Can you work these out from the model? Positions are in its coordinate system, mm. Give positions to 0.01 mm unless a question says otherwise; leave off trailing zeros. Order: outer loops, then holes, each group sorted by start corner. A loop starts at its lowest first (then second) coordinate and runs counter-clockwise, first axis right, second up.
Item 1: I want a section at B-B, the plane z = 12. Write out the boundary of the cut face in (x, y), then the cut area to 3 significant figures.
Item 2: I want a section at C-C, the plane y = 1.4. Count the separate pieces of the cut face and the enclosed holes in it, then the cut area to 3 significant figures.
Item 3: If I drill on line 1 along X through (y, z) = (2.1, -27.88); line 2 along X through (y, z) = (3.8, -28.5); line 3 along Z through (x, y) = (26.5, 3.15), over which ranges is the centre line in solid material (lowest first)?
Item 4: I want a section at A-A, the plane x = -2.5. Write out the boundary of the cut face in (y, z).
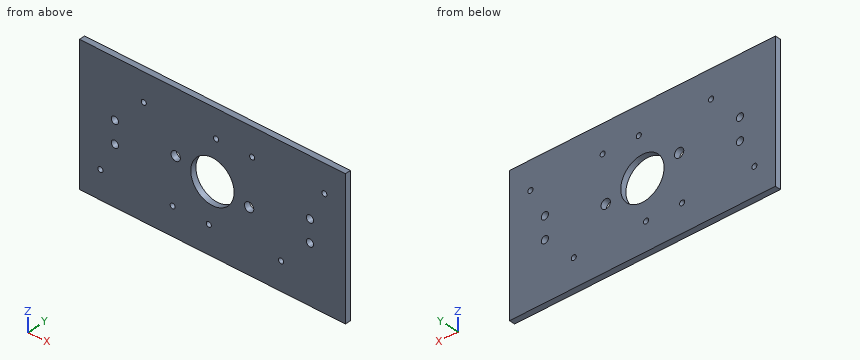
```python
from build123d import *

# Parameters (mm, degrees)
SKETCH1_W           = 184
SKETCH1_H           = 94
SKETCH1_R           = 15
SKETCH1_R_2         = 1.75
SKETCH1_R_3         = 3.225
SKETCH1_R_4         = 2.5
BOSS_EXTRUDE1_DEPTH = 4


with BuildPart() as part:
    # Sketch1 → Boss-Extrude1 (new body)
    with BuildSketch(Plane(origin=(0, 0, 0), x_dir=(1, 0, 0), z_dir=(0, 1, 0))):
        Rectangle(SKETCH1_W, SKETCH1_H)
        with Locations(Location((0, 0, 0), (0, 0, 270))):
            Circle(SKETCH1_R, mode=Mode.SUBTRACT)
        with Locations(Location((-2.5, 27.88, 0), (0, 0, 270))):
            Circle(SKETCH1_R_2, mode=Mode.SUBTRACT)
        with Locations(Location((-27.5, 27.88, 0), (0, 0, 270))):
            Circle(SKETCH1_R_2, mode=Mode.SUBTRACT)
        with Locations(Location((47.5, 27.88, 0), (0, 0, 270))):
            Circle(SKETCH1_R_2, mode=Mode.SUBTRACT)
        with Locations(Location((-77.5, 27.88, 0), (0, 0, 270))):
            Circle(SKETCH1_R_2, mode=Mode.SUBTRACT)
        with Locations(Location((25.4, 4.36, 0), (0, 0, 270))):
            Circle(SKETCH1_R_3, mode=Mode.SUBTRACT)
        with Locations(Location((-67.5, 7.5, 0), (0, 0, 270))):
            Circle(SKETCH1_R_4, mode=Mode.SUBTRACT)
        with Locations(Location((67.5, 7.5, 0), (0, 0, 270))):
            Circle(SKETCH1_R_4, mode=Mode.SUBTRACT)
        with Locations(Location((77.5, -27.88, 0), (0, 0, 270))):
            Circle(SKETCH1_R_2, mode=Mode.SUBTRACT)
        with Locations(Location((27.5, -27.88, 0), (0, 0, 270))):
            Circle(SKETCH1_R_2, mode=Mode.SUBTRACT)
        with Locations(Location((2.5, -27.88, 0), (0, 0, 270))):
            Circle(SKETCH1_R_2, mode=Mode.SUBTRACT)
        with Locations(Location((-47.5, -27.88, 0), (0, 0, 270))):
            Circle(SKETCH1_R_2, mode=Mode.SUBTRACT)
        with Locations(Location((-25.4, -4.36, 0), (0, 0, 270))):
            Circle(SKETCH1_R_3, mode=Mode.SUBTRACT)
        with Locations(Location((-67.5, -7.5, 0), (0, 0, 270))):
            Circle(SKETCH1_R_4, mode=Mode.SUBTRACT)
        with Locations(Location((67.5, -7.5, 0), (0, 0, 270))):
            Circle(SKETCH1_R_4, mode=Mode.SUBTRACT)
    extrude(amount=BOSS_EXTRUDE1_DEPTH)


solid = part.part
```
Results list:
1. outline: (-92, 0) - (-9, 0) - (-9, 4) - (-92, 4) - close; (9, 0) - (92, 0) - (92, 4) - (9, 4) - close
1. area: 664 mm2
2. separate pieces: 1
2. enclosed holes: 15
2. area: 16,400 mm2
3. line 1: x = -92 to -79.25, -75.75 to -29.25, -25.75 to -4.25, -0.75 to 45.75, 49.25 to 92
3. line 2: x = -92 to -79.14, -75.86 to -29.14, -25.86 to -4.14, -0.86 to 45.86, 49.14 to 92
3. line 3: z = -47 to -7.39, -1.33 to 26.44, 29.32 to 47
4. outline: (0, -47) - (4, -47) - (4, -29.63) - (0, -29.63) - close; (0, -26.13) - (4, -26.13) - (4, -14.79) - (0, -14.79) - close; (0, 14.79) - (4, 14.79) - (4, 47) - (0, 47) - close
